Geometry check sheet. Reference: drawing and pictorial views, mm from the part's lowest x, y, z. A direction names the side the tool comes from. Round coordinates to 2 decimals unless told otherwise and drop trailing zeros. Write each loop counter-clockwise with the first axis right and the second up, starting at its lowest first coordinate (ties: lowest second). Pieces come first, ordered by that corner, then holes. Notation, with made-up numbers: M 53.5,-19 L 77.5,-19 A27 ccw 77.5,2 Z; hole C 77.5,33.25 d3. An arc over 180 degrees is marked long. One line per question, with ' | ' between items.
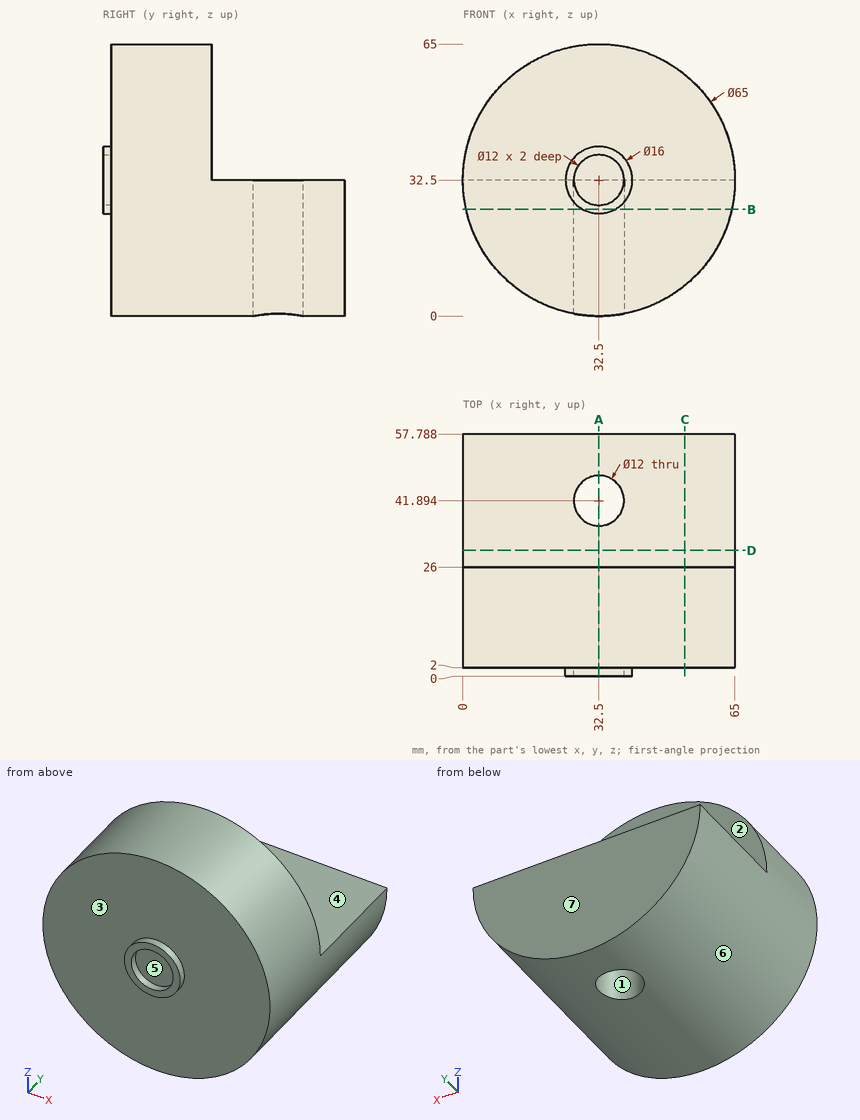
1. Section check B-B, the plane z = 25.5. Record the cut outline in (x, y).
Results:
outline: M 0.76,2 L 28.63,2 L 28.63,0 L 36.37,0 L 36.37,2 L 64.24,2 L 64.24,57.79 L 0.76,57.79 Z; hole C 32.5,41.89 d12
2. Section check D-D, the plane y = 30. Record the cut outline in (x, z), then the cut area to 3 significant figures.
Results:
outline: M 0,32.5 A32.5 ccw 65,32.5 Z | area: 1,660 mm2
3. Section check A-A, the plane x = 32.5. Record the cut outline in (y, z).
Results:
outline: M 0,24.5 L 2,24.5 L 2,0 L 35.89,0 L 35.89,32.5 L 26,32.5 L 26,65 L 2,65 L 2,40.5 L 0,40.5 L 0,38.5 L 2,38.5 L 2,26.5 L 0,26.5 Z; M 47.89,0 L 57.79,0 L 57.79,32.5 L 47.89,32.5 Z
4. Tool access check on the marked faces 1, 2 and 3. Record the directions out of +Z, -Z, +X, -X, +Y, -Y that give a thin tool (end or side, any length) a straight path to the whole face; none if there is none.
Results:
face 1: +Z, -Z | face 2: +Z, +X, -X, +Y | face 3: -Y
5. Mould release check, pull along Z, two halves, no side actions. Record for the marked faces 4, 5, 6 and 7: pulls with the +Z half, pulls with the -Z half, needs draft (parallel to the pull), parting line crosses it, or undercut.
Results:
face 4: pulls with the +Z half | face 5: undercut | face 6: parting line crosses it | face 7: needs draft
6. Section check C-C, the plane x = 53. Record the cut outline in (y, z), then the cut area to 3 significant figures.
Results:
outline: M 2,7.28 L 57.79,7.28 L 57.79,32.5 L 26,32.5 L 26,57.72 L 2,57.72 Z | area: 2,010 mm2
7. Go/stop test with flat-tipped pins: P1, Ø9.5, axis at x = 39, y = 42.5, coming from the +Z side; P2, Ø19.5, axis at x = 22.5, z = 45, coming from the -Y side; P3, Ø16, axis at x = 26.5, z = 45.5, coming from the +Y side; P4, Ø4, axis at y = 34, z = 21.5, coming from the +X side. Record where each tip stops, or that it passes through.
Results:
P1: stops at z = 32.5 | P2: stops at y = 0 | P3: stops at y = 26 | P4: stops at x = 63.73
8. Thickness scan on line 1 (Y direction, x = 38, z = 40); line 2 (Y direction, x = 40, z = 22); line 3 (X direction, y = 45.5, z = 22.5). Record the ranges inside material, lowest first.
Results:
line 1: y = 2 to 26 | line 2: y = 2 to 57.79 | line 3: x = 1.58 to 27.7, 37.3 to 63.42
